from build123d import *

# Parameters (mm, degrees)
PARED_START                  = -39.75
SK_PARED_W                   = 100
SK_PARED_H                   = 92
PARED_DEPTH                  = 10
CABEZA_START                 = -39.75
SK_CABEZA_R                  = 50
CABEZA_DEPTH                 = 10
ASIENTO_1MM_START            = -29.75
SK_ASIENTO_1MM_R             = 42
SK_ASIENTO_1MM_R_2           = 29
ASIENTO_1MM_DEPTH            = 1
PASO_BOSS_J2_START           = -39.75
SK_PASO_BOSS_J2_R            = 29
PASO_BOSS_J2_DEPTH           = 11
PASANTES_M3_ESTATOR_J2_START = -39.75
SK_PASANTES_M3_ESTATOR_J2_R  = 1.7
PASANTES_M3_ESTATOR_J2_DEPTH = 11
PASANTES_M4_ANGULOS_START    = -39.75
SK_PASANTES_M4_ANGULOS_R     = 2.25
PASANTES_M4_ANGULOS_DEPTH    = 10


with BuildPart() as part:
    # Sk_Pared → Pared (new body)
    with BuildSketch(Plane(origin=(0, 0, 0), x_dir=(1, 0, 0), z_dir=(0, 1, 0)).offset(PARED_START)):
        with Locations((0, -124)):
            Rectangle(SK_PARED_W, SK_PARED_H)
    extrude(amount=PARED_DEPTH)

    # Sk_Cabeza → Cabeza (add)
    with BuildSketch(Plane(origin=(0, 0, 0), x_dir=(1, 0, 0), z_dir=(0, 1, 0)).offset(CABEZA_START)):
        with Locations((0, -170)):
            Circle(SK_CABEZA_R)
    extrude(amount=CABEZA_DEPTH)

    # Sk_Asiento_1mm → Asiento_1mm (add)
    with BuildSketch(Plane(origin=(0, 0, 0), x_dir=(1, 0, 0), z_dir=(0, 1, 0)).offset(ASIENTO_1MM_START)):
        with Locations(Location((0, -170, 0), (0, 0, 270))):
            Circle(SK_ASIENTO_1MM_R)
        with Locations(Location((0, -170, 0), (0, 0, 270))):
            Circle(SK_ASIENTO_1MM_R_2, mode=Mode.SUBTRACT)
    extrude(amount=ASIENTO_1MM_DEPTH)

    # Sk_Paso_boss_J2 → Paso_boss_J2 (cut)
    with BuildSketch(Plane(origin=(0, 0, 0), x_dir=(1, 0, 0), z_dir=(0, 1, 0)).offset(PASO_BOSS_J2_START)):
        with Locations(Location((0, -170, 0), (0, 0, 270))):
            Circle(SK_PASO_BOSS_J2_R)
    extrude(amount=PASO_BOSS_J2_DEPTH, mode=Mode.SUBTRACT)

    # Sk_Pasantes_M3_estator_J2 → Pasantes_M3_estator_J2 (cut)
    with BuildSketch(Plane(origin=(0, 0, 0), x_dir=(1, 0, 0), z_dir=(0, 1, 0)).offset(PASANTES_M3_ESTATOR_J2_START)):
        with Locations(Location((37, -170, 0), (0, 0, 270))):
            Circle(SK_PASANTES_M3_ESTATOR_J2_R)
        with Locations(Location((26.162950904, -196.162950904, 0), (0, 0, 270))):
            Circle(SK_PASANTES_M3_ESTATOR_J2_R)
        with Locations(Location((0, -207, 0), (0, 0, 270))):
            Circle(SK_PASANTES_M3_ESTATOR_J2_R)
        with Locations(Location((-26.162950904, -196.162950904, 0), (0, 0, 270))):
            Circle(SK_PASANTES_M3_ESTATOR_J2_R)
        with Locations(Location((-37, -170, 0), (0, 0, 270))):
            Circle(SK_PASANTES_M3_ESTATOR_J2_R)
        with Locations(Location((-26.162950904, -143.837049096, 0), (0, 0, 270))):
            Circle(SK_PASANTES_M3_ESTATOR_J2_R)
        with Locations(Location((0, -133, 0), (0, 0, 270))):
            Circle(SK_PASANTES_M3_ESTATOR_J2_R)
        with Locations(Location((26.162950904, -143.837049096, 0), (0, 0, 270))):
            Circle(SK_PASANTES_M3_ESTATOR_J2_R)
    extrude(amount=PASANTES_M3_ESTATOR_J2_DEPTH, mode=Mode.SUBTRACT)

    # Sk_Pasantes_M4_angulos → Pasantes_M4_angulos (cut)
    with BuildSketch(Plane(origin=(0, 0, 0), x_dir=(1, 0, 0), z_dir=(0, 1, 0)).offset(PASANTES_M4_ANGULOS_START)):
        with Locations(Location((-21, -89.11, 0), (0, 0, 270))):
            Circle(SK_PASANTES_M4_ANGULOS_R)
        with Locations(Location((21, -89.11, 0), (0, 0, 270))):
            Circle(SK_PASANTES_M4_ANGULOS_R)
    extrude(amount=PASANTES_M4_ANGULOS_DEPTH, mode=Mode.SUBTRACT)


solid = part.part
The model under review builds one solid part; all positions refer to its coordinate system, in mm. Round coordinates to 2 decimals unless told otherwise and drop trailing zeros. Loops run counter-clockwise (first coordinate to the right, second up) from the corner with the lowest first, then second, coordinate; pieces in that order, holes last. Notation, with made-up numbers: (4.5, 21) -> (33.5, 21) arc R30 ccw to (33.5, 51) -> close; hole circle Ø7 at (46, -39). An arc over 180 degrees is marked (long way). Write item = value, one per line. Start each with the question number.
Item 1: Take a section at C-C on x = 37. Give the boundary of the cut face in (y, z).
Item 2: Take a section at A-A on x = 0. Give the boundary of the cut face in (y, z).
Item 3: Insertion check: pin 1 (10 mm diameter, centred on x = -21.5, z = 156.5, fed in from +Y); pin 2 (1 mm diameter, centred on x = 34.5, y = -32.5, fed in from +Z); pin 3 (3 mm diameter, centred on x = 36, y = -34.5, fed in from +Z). Each pin has a flat end and moves straight along its axis. Give the tip position at first contact, or say it passes through.
Item 4: Mouldability with a two-part tool opening along X and no side actions: class faces 1 (the cylindrical face through (25.129, -34.327, 142.488)), 2 (the cylindrical face through (1.85, -29.26, 128.04)), 3 (the cylindrical face through (1.433, -34.327, 133.914)), 4 (the flat face through (-1, -35, 78)) as released by +X, released by -X, zero draft, split by the parting line, or undercut.
Item 5: Take a section at D-D on z = 163.5. Give the boundary of the cut face in (x, y).
Item 6: To check wall thickness, follow L1, parallel to X at y = -37, z = 89.11; L2, parallel to X at y = -35, z = 170; L3, parallel to Z at x = 25.5, y = -34.5. State the ranges of each line that lie inside material, in increasing order.
Item 7: Take a section at B-B on z = 89.11. Give the boundary of the cut face in (x, y), plus the area to 3 significant figures.
Result:
q1.outline = (-39.75, 78) -> (-29.75, 78) -> (-29.75, 150.13) -> (-28.75, 150.13) -> (-28.75, 168.3) -> (-39.75, 168.3) -> close; (-39.75, 171.7) -> (-28.75, 171.7) -> (-28.75, 189.87) -> (-29.75, 189.87) -> (-29.75, 203.63) -> (-39.75, 203.63) -> close
q2.outline = (-39.75, 78) -> (-29.75, 78) -> (-29.75, 128) -> (-28.75, 128) -> (-28.75, 131.3) -> (-39.75, 131.3) -> close; (-39.75, 134.7) -> (-28.75, 134.7) -> (-28.75, 141) -> (-39.75, 141) -> close; (-39.75, 199) -> (-28.75, 199) -> (-28.75, 205.3) -> (-39.75, 205.3) -> close; (-39.75, 208.7) -> (-28.75, 208.7) -> (-28.75, 212) -> (-29.75, 212) -> (-29.75, 220) -> (-39.75, 220) -> close
q3.pin_1 = -28.75
q3.pin_2 = 206.66
q3.pin_3 = 206.19
q4.face_1 = undercut
q4.face_2 = split by the parting line
q4.face_3 = undercut
q4.face_4 = zero draft
q5.outline = (-50, -39.75) -> (-28.26, -39.75) -> (-28.26, -28.75) -> (-41.49, -28.75) -> (-41.49, -29.75) -> (-50, -29.75) -> close; (28.26, -39.75) -> (50, -39.75) -> (50, -29.75) -> (41.49, -29.75) -> (41.49, -28.75) -> (28.26, -28.75) -> close
q6.L1 = -50 to -23.25, -18.75 to 18.75, 23.25 to 50
q6.L2 = -50 to -38.7, -35.3 to -29, 29 to 35.3, 38.7 to 50
q6.L3 = 78 to 142.27, 145.4 to 156.19, 183.81 to 194.6, 197.73 to 213.01
q7.outline = (-50, -39.75) -> (-23.25, -39.75) -> (-23.25, -29.75) -> (-50, -29.75) -> close; (-18.75, -39.75) -> (18.75, -39.75) -> (18.75, -29.75) -> (-18.75, -29.75) -> close; (23.25, -39.75) -> (50, -39.75) -> (50, -29.75) -> (23.25, -29.75) -> close
q7.area = 910 mm²
